Input: part model. Units: mm. Frame: model coordinates. A direction names the side the tool comes from. Round coordinates to 2 decimals unless told otherwise and drop trailing zeros. Order: outer loops, then holes, each group sorted by start corner. A loop starts at its lowest first (then second) coordinate and runs counter-clockwise, first axis right, second up. Notation, with made-up numbers: (54, 40) -> (96, 40) arc R14 cw to (96, 57) -> close; hole circle Ø9 at (83, 54.5). An arc over 180 degrees is marked (long way). Answer as CSV lines item,"result". Start each with the question number.
1) Line query: L1, parallel to X at y = 5.5, z = 8.25; L2, parallel to X at y = 1.5, z = 4; L3, parallel to Z at x = -3.5, y = 6.75. Output: solid intervals per line, ascending.
2) Section query C-C, the plane z = -1.5. Output: boundary loops of the cut face in (x, y), and give its area (3 significant figures).
3) Access query for faces 4 (the face through (-16, 4, 0)), 5 (the face through (7.863, 3.944, 7.692)), 6 (the face through (-17, 0, 3)), 7 (the face through (10, 4, 0)), 8 (the face through (-43, 4, 0)). Directions: +Z, -Z, +X, -X, +Y, -Y. A direction counts if a zero-diameter tool reaches every point of the face in a straight line with its end or side. Return the directions, or none.
4) Section query D-D, the plane x = -14. Output: boundary loops of the cut face in (y, z).
5) Section query A-A, the plane y = 3. Output: boundary loops of the cut face in (x, z), and give its area (3 significant figures).
6) Mould query, pull axis Z, two halves, no side actions, for faces 1 (the face through (-24.93, 3.94, -7.69)), 2 (the face through (-26.225, 3.944, 6.151)), 3 (the face through (0, 4, -10)). Classes: +Z half, -Z half, draft (parallel to the pull), parting line (faces both ways), or undercut.
7) Section query B-B, the plane x = -6.5. Output: boundary loops of the cut face in (y, z), and give its area (3 significant figures).
8) First-contact query: P1, Ø1.6, axis at y = 5.5, z = -10, coming from the -X side; P2, Ø0.6, axis at x = -43, y = 2.5, coming from the -Z side; P3, Ø1.5, axis at x = -37, y = 5.5, coming from the +Z side; P4, Ø3, axis at y = 5, z = -0.5, coming from the -X side. Flat tips, straight axial feed; report the tip coordinate or a pass-through.
```python
from build123d import *

# Parameters (mm, degrees)
BOSS_EXTRUDE1_DEPTH = 8


with BuildPart() as part:
    # Sketch1 → Boss-Extrude1 (new body)
    with BuildSketch(Plane(origin=(0, 0, 0), x_dir=(1, 0, 0), z_dir=(0, 1, 0))):
        with BuildLine():
            ThreePointArc((-43.795204124, 0), (-25.017029531, -7.778174593), (-32.795204124, 11))
            Line((-32.795204124, 11), (-32.795204124, 9))
            ThreePointArc((-32.795204124, 9), (-26.431243094, -6.363961031), (-41.795204124, 0))
            Line((-41.795204124, 0), (-43.795204124, 0))
        make_face()
        with BuildLine():
            Line((-16.397602062, -11), (-16.397602062, 0))
            Line((-16.397602062, 0), (-21.795204124, 0))
            ThreePointArc((-21.795204124, 0), (-25.017029531, -7.778174593), (-32.795204124, -11))
            Line((-32.795204124, -11), (-16.397602062, -11))
        make_face()
        with BuildLine():
            ThreePointArc((0, -11), (-7.778174593, -7.778174593), (-11, 0))
            Line((-11, 0), (-16.397602062, 0))
            Line((-16.397602062, 0), (-16.397602062, -11))
            Line((-16.397602062, -11), (0, -11))
        make_face()
        with BuildLine():
            ThreePointArc((11, 0), (-7.778174593, -7.778174593), (0, 11))
            Line((0, 11), (0, 9))
            ThreePointArc((0, 9), (-6.363961031, -6.363961031), (9, 0))
            Line((9, 0), (11, 0))
        make_face()
    extrude(amount=BOSS_EXTRUDE1_DEPTH)


solid = part.part
```
Findings:
1,L1,"x = -40.07 to -36.39, -29.2 to -3.6, 3.6 to 7.28"
1,L2,"x = -43.04 to -40.86, -24.73 to -8.06, 8.06 to 10.25"
1,L3,"z = -10.43 to -8.29, 8.29 to 11"
2,outline,"(-23.92, 0) -> (-21.9, 0) -> (-21.9, 8) -> (-23.92, 8) -> close; (-10.9, 0) -> (-8.87, 0) -> (-8.87, 8) -> (-10.9, 8) -> close"
2,area,"32.4 mm^2"
3,face 4,"-Z, +Y, -Y"
3,face 5,"+Z, +X, +Y, -Y"
3,face 6,"+Z, -Z, +X, -X, -Y"
3,face 7,"-Z, +X, +Y, -Y"
3,face 8,"-Z, -X, +Y, -Y"
4,outline,"(0, 0) -> (8, 0) -> (8, 11) -> (0, 11) -> close"
5,outline,"(-43.8, 0) -> (-41.8, 0) arc R9 cw (long way) to (-32.8, -9) -> (-32.8, -11) arc R11 ccw to (-21.8, 0) -> (-11, 0) arc R11 ccw to (0, -11) -> (0, -9) arc R9 cw (long way) to (9, 0) -> (11, 0) arc R11 ccw to (0, 11) -> (-32.8, 11) arc R11 ccw to start"
5,area,"359 mm^2"
6,face 1,"-Z half"
6,face 2,"undercut"
6,face 3,"draft"
7,outline,"(0, -8.87) -> (8, -8.87) -> (8, -6.22) -> (0, -6.22) -> close; (0, 6.22) -> (8, 6.22) -> (8, 11) -> (0, 11) -> close"
7,area,"59.4 mm^2"
8,P1,"stops at x = -32.8"
8,P2,"stops at z = 0"
8,P3,"stops at z = 10.44"
8,P4,"stops at x = -43.8"
